Could you check a few things on this model? Use its own coordinates, in mm. A direction names the side the tool comes from. Round coordinates to 2 decimals unless told otherwise and drop trailing zeros. Write each loop counter-clockwise with the first axis right and the second up, starting at its lowest first coordinate (ties: lowest second). Pieces come first, ordered by that corner, then holes. Notation, with made-up numbers: (86, -33.5) - (125, -33.5) arc R17 cw to (125, -12.5) - close; hole circle Ø3 at (-16.5, 56). An arc over 180 degrees is marked (long way). Write each question's results on one line, items separated by ' | '. Start each with the question number.
(1) Imagine slicing it at D-D on y = 59. Write out the boundary of the cut face in (x, z), then the cut area to 3 significant figures.
(2) Thinking about a two-plate mould opening in Y: for faces 6 (the cylindrical face through (-20.44, 69, 1.48)), 7 (the cylindrical face through (-25.78, 61.74, 1.48)), 8 (the cylindrical face through (-84.26, 66.02, -12.57)), which applies, +Y half, -Y half, draft (parallel to the pull), parting line (faces both ways), or undercut?
(3) Imagine slicing it at B-B on z = -25. Write out the boundary of the cut face in (x, y).
(4) For P1, Ø5, axis at x = -68.5, y = 66, coming from the +Z side; P2, Ø1.2, axis at x = -29.98, y = 59, coming from the +Z side; P3, Ø3.5, axis at x = -34.93, y = 61.05, coming from the -Z side; P4, Ø0.9, axis at x = -29.5, y = 66, coming from the +Z side, each with a flat end and sliding along its axis, tell me the tip position at first contact or that it passes through.
(5) Imagine slicing it at C-C on z = -19. Write out the boundary of the cut face in (x, y).
(6) Please list where these lines run through material, in increasing order: line 1 (X direction, y = 66.5, z = -25); line 2 (X direction, y = 66, z = 1.35); line 3 (Z direction, x = -26.5, y = 70.75). Write a range as [from, to].
(7) On a 3-axis mill with a long thin cutter (end or side, diameter ignored), from which of +Z, -Z, +X, -X, +Y, -Y can I reach the whole of each face in a straight line? I mean faces 1 (the flat face through (-37, 66, 0)), 2 (the flat face through (-68, 66, -37)), 3 (the flat face through (-67, 66, -12)), 4 (the flat face through (-76.397, 66, -25)), 5 (the flat face through (-30, 61, 0)). Say none if no direction works.
(8) Imagine slicing it at A-A on x = -60. Write out the boundary of the cut face in (y, z), then the cut area to 3 significant figures.
```python
from build123d import *

# Parameters (mm, degrees)
SKETCH_1_R               = 10
SKETCH_1_R_2             = 1.02
SKETCH_1_R_3             = 1.5
EXTRUDE_1_DEPTH          = 3
SKETCH_2_R               = 5
EXTRUDE_2_DEPTH          = 1
CUT_EXTRUDE_1_DEPTH      = 10
CUT_EXTRUDE_1_DEPTH_BACK = 0.5
SKETCH_3_R               = 3
SKETCH_4_R               = 1.5
CUT_EXTRUDE_2_DEPTH      = 8.5
CUT_EXTRUDE_START        = -10
SKETCH_5_R               = 3
CUT_EXTRUDE_3_DEPTH      = 10
EXTRUDE_3_DEPTH          = 50
SKETCH_7_W               = 26.150152834
SKETCH_7_H               = 10
SKETCH_7_R               = 1.5
SKETCH_7_R_2             = 3
SKETCH_7_R_3             = 2.2
CUT_EXTRUDE_8_DEPTH      = 50
SKETCH_9_W               = 3.765706055
SKETCH_9_H               = 11.940159279
CUT_EXTRUDE_9_DEPTH      = 50


with BuildPart() as part:
    # ｽｹｯﾁ1 → ﾎﾞｽ - 押し出し1 (new body)
    with BuildSketch(Plane.XY):
        with Locations((-29.978703949, 66)):
            Circle(SKETCH_1_R)
        with Locations((-25.028956481, 61.050252532)):
            Circle(SKETCH_1_R_2, mode=Mode.SUBTRACT)
        with Locations((-29.978703949, 59)):
            Circle(SKETCH_1_R_2, mode=Mode.SUBTRACT)
        with Locations((-34.928451418, 61.050252532)):
            Circle(SKETCH_1_R_2, mode=Mode.SUBTRACT)
        with Locations((-36.978703949, 66)):
            Circle(SKETCH_1_R_2, mode=Mode.SUBTRACT)
        with Locations((-34.928451418, 70.949747468)):
            Circle(SKETCH_1_R_2, mode=Mode.SUBTRACT)
        with Locations((-29.978703949, 73)):
            Circle(SKETCH_1_R_2, mode=Mode.SUBTRACT)
        with Locations((-25.028956481, 70.949747468)):
            Circle(SKETCH_1_R_2, mode=Mode.SUBTRACT)
        with Locations((-22.978703949, 66)):
            Circle(SKETCH_1_R_2, mode=Mode.SUBTRACT)
        with Locations((-29.978703949, 66)):
            Circle(SKETCH_1_R_3, mode=Mode.SUBTRACT)
    extrude(amount=EXTRUDE_1_DEPTH)

    # ｽｹｯﾁ2 → ﾎﾞｽ - 押し出し2 (add)
    with BuildSketch(Plane.XY.offset(3)):
        with Locations((-29.978703949, 66)):
            Circle(SKETCH_2_R)
    extrude(amount=EXTRUDE_2_DEPTH)

    # ｽｹｯﾁ3 → ｶｯﾄ - 押し出し1 (cut, two sides: drawn at the far end of the back side and taken through both)
    with BuildSketch(Plane(origin=(0, 0, 3), x_dir=(-1, 0, 0), z_dir=(0, 0, -1)).offset(-CUT_EXTRUDE_1_DEPTH_BACK)):
        with Locations(Location((29.978703949, 66, 0), (0, 0, 180))):
            Circle(SKETCH_3_R)
    extrude(amount=CUT_EXTRUDE_1_DEPTH + CUT_EXTRUDE_1_DEPTH_BACK, mode=Mode.SUBTRACT)

    # ｽｹｯﾁ4 → ｶｯﾄ - 押し出し2 (cut)
    with BuildSketch(Plane(origin=(0, 0, 3.5), x_dir=(-1, 0, 0), z_dir=(0, 0, -1))):
        with Locations((29.978703949, 66)):
            Circle(SKETCH_4_R)
    extrude(amount=-CUT_EXTRUDE_2_DEPTH, mode=Mode.SUBTRACT)

    # ｽｹｯﾁ5 → ｶｯﾄ - 押し出し3 (cut)
    with BuildSketch(Plane(origin=(0, 0, 0), x_dir=(-1, 0, 0), z_dir=(0, 0, -1)).offset(CUT_EXTRUDE_START)):
        with Locations(Location((29.978703949, 66, 0), (0, 0, 180))):
            Circle(SKETCH_5_R)
    extrude(amount=CUT_EXTRUDE_3_DEPTH, mode=Mode.SUBTRACT)

    # ｽｹｯﾁ6 → ﾎﾞｽ - 押し出し3 (add)
    with BuildSketch(Plane(origin=(0, 0, 0), x_dir=(-1, 0, 0), z_dir=(0, 0, -1))):
        Polygon((29.978703949, 64.5), (89.978703949, 64.5), (89.978703949, 67.5), (29.978703949, 67.5), (7.978703949, 67.5), (7.978703949, 64.5), align=None)
    extrude(amount=EXTRUDE_3_DEPTH)

    # ｽｹｯﾁ7 → ｶｯﾄ - 押し出し8 (cut)
    with BuildSketch(Plane(origin=(0, 67.5, 0), x_dir=(1, 0, 0), z_dir=(0, 1, 0))):
        with BuildLine():
            Line((-100.145182103, -3.51175574), (-39.985484803, 0))
            Line((-39.985484803, 0), (-51.974034344, 12))
            Line((-51.974034344, 12), (-82.864348742, 12))
            ThreePointArc((-82.864348742, 12), (-84.278562304, 12.585786438), (-84.864348742, 14))
            Line((-84.864348742, 14), (-84.864348742, 35))
            ThreePointArc((-84.864348742, 35), (-84.278562304, 36.414213562), (-82.864348742, 37))
            Line((-82.864348742, 37), (-51.974034344, 37))
            Line((-51.974034344, 37), (-40.543200867, 48.912989303))
            ThreePointArc((-40.543200867, 48.912989303), (-39.734398684, 49.588968373), (-38.763748554, 50))
            Line((-38.763748554, 50), (-38.44069987, 54.873631325))
            Line((-38.44069987, 54.873631325), (-103.044452856, 56.708369205))
            Line((-103.044452856, 56.708369205), (-100.145182103, -3.51175574))
        make_face()
        with BuildLine():
            Line((-19.971923095, 56.200079543), (-21.193659345, 50))
            ThreePointArc((-21.193659345, 50), (-20.151061293, 49.706748166), (-19.414207032, 48.912989303))
            Line((-19.414207032, 48.912989303), (-9.074178765, 28.759864671))
            ThreePointArc((-9.074178765, 28.759864671), (-7.978703949, 25), (-9.074178765, 21.240135329))
            Line((-9.074178765, 21.240135329), (-19.971923095, 0))
            Line((-19.971923095, 0), (8.860799546, -5.1085516))
            Line((8.860799546, -5.1085516), (11.142393262, 56.200079543))
            Line((11.142393262, 56.200079543), (-19.971923095, 56.200079543))
        make_face()
        with Locations((-63.322025342, 25)):
            Rectangle(SKETCH_7_W, SKETCH_7_H)
        with Locations(Location((-14.978703949, 25, 0), (0, 0, 270))):
            Circle(SKETCH_7_R)
        with Locations(Location((-22.387170595, 46.444557629, 0), (0, 0, 270))):
            Circle(SKETCH_7_R)
        with Locations(Location((-37.570237303, 46.444557629, 0), (0, 0, 270))):
            Circle(SKETCH_7_R)
        with Locations(Location((-44.978703949, 25, 0), (0, 0, 270))):
            Circle(SKETCH_7_R_2)
        with Locations(Location((-79.978703949, 30, 0), (0, 0, 270))):
            Circle(SKETCH_7_R_3)
        with Locations(Location((-79.978703949, 20, 0), (0, 0, 270))):
            Circle(SKETCH_7_R_3)
        with Locations(Location((-29.978703949, 30, 0), (0, 0, 270))):
            Circle(SKETCH_7_R_3)
        with Locations(Location((-29.978703949, 20, 0), (0, 0, 270))):
            Circle(SKETCH_7_R_3)
    extrude(amount=-CUT_EXTRUDE_8_DEPTH, mode=Mode.SUBTRACT)

    # ｽｹｯﾁ9 → ｶｯﾄ - 押し出し9 (cut)
    with BuildSketch(Plane(origin=(0, 0, 0), x_dir=(0, 0, -1), z_dir=(1, 0, 0))):
        with Locations((-4.882853028, 66.970079639)):
            Rectangle(SKETCH_9_W, SKETCH_9_H)
    extrude(amount=-CUT_EXTRUDE_9_DEPTH, mode=Mode.SUBTRACT)


solid = part.part
```
Response:
1) outline: (-37.12, 0) - (-31, 0) - (-31, 3) - (-37.12, 3) - close; (-28.96, 0) - (-22.84, 0) - (-22.84, 3) - (-28.96, 3) - close | area: 36.7 mm²
2) face 6: parting line | face 7: undercut | face 8: draft
3) outline: (-84.86, 64.5) - (-76.4, 64.5) - (-76.4, 67.5) - (-84.86, 67.5) - close; (-50.25, 64.5) - (-47.98, 64.5) - (-47.98, 67.5) - (-50.25, 67.5) - close; (-41.98, 64.5) - (-16.48, 64.5) - (-16.48, 67.5) - (-41.98, 67.5) - close; (-13.48, 64.5) - (-7.98, 64.5) - (-7.98, 67.5) - (-13.48, 67.5) - close
4) P1: z = -12 | P2: through | P3: z = 0 | P4: z = 0
5) outline: (-84.86, 64.5) - (-81.94, 64.5) - (-81.94, 67.5) - (-84.86, 67.5) - close; (-78.02, 64.5) - (-31.94, 64.5) - (-31.94, 67.5) - (-78.02, 67.5) - close; (-28.02, 64.5) - (-10.22, 64.5) - (-10.22, 67.5) - (-28.02, 67.5) - close
6) line 1: [-84.86, -76.4], [-50.25, -47.98], [-41.98, -16.48], [-13.48, -7.98] | line 2: [-39.98, -38], [-35.96, -32.98], [-26.98, -24], [-21.96, -19.98] | line 3: [0, 3]
7) face 1: +Z | face 2: -Z, -X, +Y, -Y | face 3: +Z, -X, +Y, -Y | face 4: +Y, -Y | face 5: -Z, +X, -X, -Y
8) outline: (64.5, -37) - (67.5, -37) - (67.5, -30) - (64.5, -30) - close; (64.5, -20) - (67.5, -20) - (67.5, -12) - (64.5, -12) - close | area: 45.0 mm²
